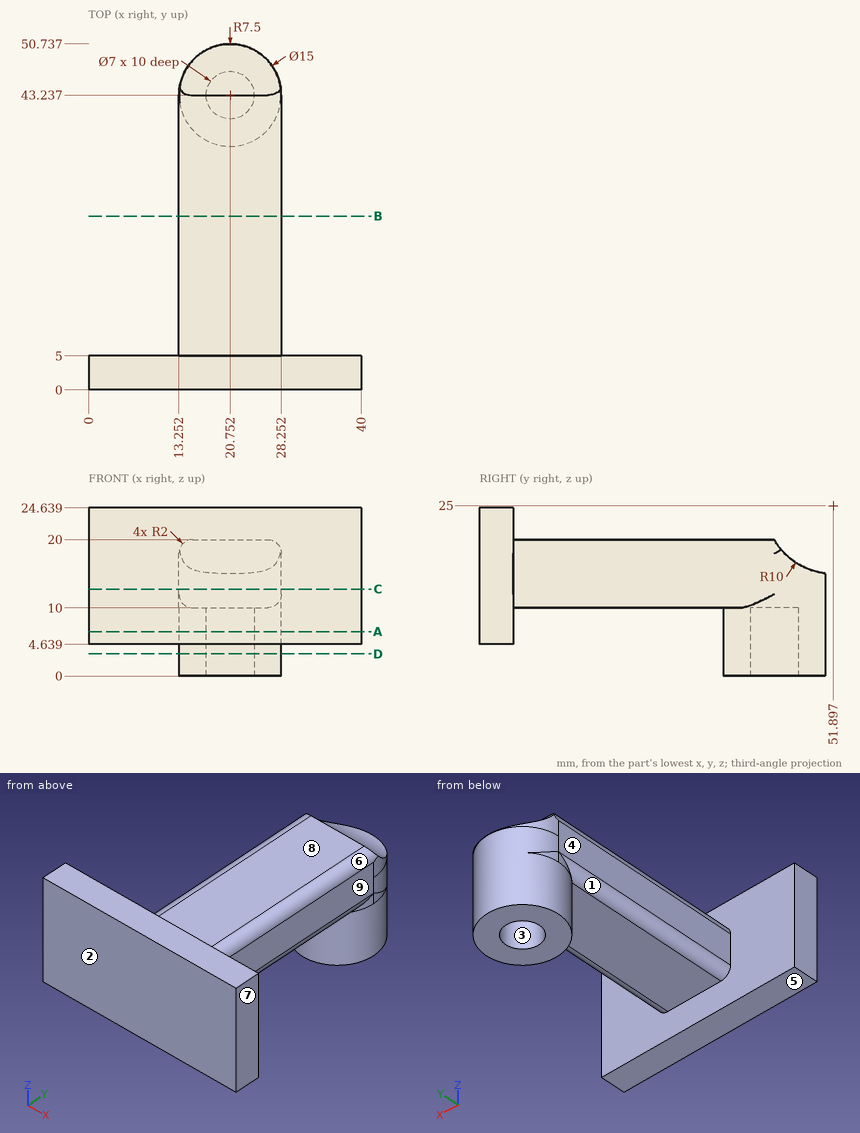
Study the drawing (mm; zero at the part's minimum x, y, z) and answer. A direction names the side the tool comes from. Give positions to 0.01 mm unless a question says otherwise; leave off trailing zeros. Order: outer loops, then holes, each group sorted by start corner. A loop starts at its lowest first (then second) coordinate and runs counter-clockwise, first axis right, second up.
1. Each of these flat-tipped pins is pushed along its axis until it touches: P1, Ø2, axis at x = 21.5, y = 43.5, coming from the -Z side; P2, Ø4, axis at y = 15, z = 9, coming from the +X side (1 decimal); P3, Ø6, axis at x = 28, z = 12, coming from the +Y side. Where does it stop, or does it pass through?
Result sheet:
P1: stops at z = 10
P2: stops at x = 28
P3: stops at y = 49.42
2. Section A-A, the plane z = 6.5 is taken. Determine the outline of the cut face in (x, y), and give its area (3 significant figures).
Result sheet:
outline: (0, 0) - (40, 0) - (40, 5) - (0, 5) - close; circle Ø15 at (20.75, 43.24); hole circle Ø7 at (20.75, 43.24)
area: 338 mm2
3. Section C-C, the plane z = 12.75 is taken. Determine the outline of the cut face in (x, y), and give its area (3 significant figures).
Result sheet:
outline: (0, 0) - (40, 0) - (40, 5) - (28.25, 5) - (28.25, 43.24) arc R7.5 ccw to (13.25, 43.24) - (13.25, 5) - (0, 5) - close
area: 862 mm2
4. Section D-D, the plane z = 3.25 is taken. Determine the outline of the cut face in (x, y).
Result sheet:
outline: circle Ø15 at (20.75, 43.24); hole circle Ø7 at (20.75, 43.24)
5. The mould has two halves that part along Y. Classify the marked faces 1, 2, 3 and 4: released by +Y, released by -Y, zero draft, split by the parting line, or undercut.
Result sheet:
face 1: undercut
face 2: released by -Y
face 3: undercut
face 4: zero draft
6. For the marked faces 5, 6, 7, 8 and 9, determine the directions among +Z, -Z, +X, -X, +Y, -Y from which every point of the face is accessible in a straight line to the end or side of a thin tool.
Result sheet:
face 5: -Z, +X, -X, -Y
face 6: +Z, +X, +Y
face 7: +Z, -Z, +X, +Y, -Y
face 8: +Z, +X, -X, +Y
face 9: +Z, -Z, +X, +Y
7. Straight lines are drawn through the part: L1, parallel to Y at x = 23, z = 7.5 (1 decimal); L2, parallel to Z at x = 23, y = 2; L3, parallel to Y at x = 10, z = 21. For each, find the intervals that lie inside material, in ascending order.
Result sheet:
L1: y = 0 to 5, 36.1 to 40.6, 45.9 to 50.4
L2: z = 4.64 to 24.64
L3: y = 0 to 5
8. Section B-B, the plane y = 25.5 is taken. Determine the outline of the cut face in (x, z), and give its area (3 significant figures).
Result sheet:
outline: (13.25, 12) arc R2 ccw to (15.25, 10) - (26.25, 10) arc R2 ccw to (28.25, 12) - (28.25, 18) arc R2 ccw to (26.25, 20) - (15.25, 20) arc R2 ccw to (13.25, 18) - close
area: 147 mm2
